```python
from build123d import *

# Parameters (mm, degrees)
F0_R     = 14.2875
F1_DEPTH = 3.175
F2_R     = 8.73125
F3_DEPTH = 1.5875
F5_DEPTH = 1.5875
F6_R     = 7.9375
F6_R_2   = 6.35
F7_DEPTH = 1.5875
F8_COUNT = 6


with BuildPart() as f1:
    # F0 (on Front) → F1 (new body)
    with BuildSketch(Plane.XZ):
        Circle(F0_R)
    extrude(amount=F1_DEPTH)

    # F2 (on face) → F3 (join)
    with BuildSketch(Plane.XZ.offset(3.175)):
        Circle(F2_R)
    extrude(amount=F3_DEPTH)

    # F4 (on face) → F5 (join)
    with BuildSketch(Plane(origin=(0, 0, 0), x_dir=(-1, 0, 0), z_dir=(0, 1, 0))):
        Polygon((11.4293787458, -1.8054905687), (12.8345400717, -0.6283202405), (12.5176613259, 1.1771703282), (10.7956212542, 1.8054905687), (9.3904599283, 0.6283202405), (9.7073386741, -1.1771703282), align=None)
    extrude(amount=F5_DEPTH)

    # F6 (on face) → F7 (join)
    with BuildSketch(Plane(origin=(0, 0, 0), x_dir=(-1, 0, 0), z_dir=(0, 1, 0))):
        Circle(F6_R)
        Circle(F6_R_2, mode=Mode.SUBTRACT)
    extrude(amount=F7_DEPTH)

    # F8: F1 ×6 about axis
    f8_axis = Axis((0, 1.5875, 0), (0, 1, 0))


with BuildPart() as f1_1:
    add(f1.part)
    for i in range(1, F8_COUNT):
        add(f1.part.rotate(f8_axis, i * 360 / F8_COUNT))


solid = f1_1.part
```
Could you check a few things on this model? Use its own coordinates, in mm. A direction names the side the tool comes from. Round coordinates to 2 decimals unless told otherwise and drop trailing zeros. Loops run counter-clockwise (first coordinate to the right, second up) from the corner with the lowest first, then second, coordinate; pieces in that order, holes last. Notation, with made-up numbers: M -25.75,-20.75 L 20.25,-20.75 A21 ccw 20.25,-9.75 Z; hole C 83.5,-35 d7. An arc over 180 degrees is marked long. Put each result on its own line as item: value.
Q1. I need wall thicknesses on probe 1 along Z at (x, y) = (0, 0.85); probe 2 along X at (y, z) = (0.8, 0); probe 3 along Y at (x, z) = (-11.75, 0.75) (1 decimal). Which ranges of each line are inside material? Lowest first, please.
Check result:
probe 1: -7.94 to -6.35, 6.35 to 7.94
probe 2: -12.72 to -9.5, -7.94 to -6.35, 6.35 to 7.94, 9.5 to 12.72
probe 3: -3.2 to 1.6
Q2. Imagine slicing it at C-C (z = 5.5). Write out the boundary of the cut face in (x, y) (1 decimal), then the cut area to 3 significant figures.
Check result:
outline: M -13.2,-3.2 L -6.8,-3.2 L -6.8,-4.8 L 6.8,-4.8 L 6.8,-3.2 L 13.2,-3.2 L 13.2,0 L 5.7,0 L 5.7,1.6 L 3.2,1.6 L 3.2,0 L -3.2,0 L -3.2,1.6 L -5.7,1.6 L -5.7,0 L -13.2,0 Z
area: 113 mm2
Q3. On a 3-axis mill with a long thin cutter (end or side, diameter ignored), from which of +Z, -Z, +X, -X, +Y, -Y can I reach the whole of each face in a straight line? I mean faces 1 (the face through (5, 0.783, -8.137)), 2 (the face through (-7, -3.175, -6)), 3 (the face through (3.99, 0.78, 9.89)), 4 (the face through (10.103, 0.783, -1.225)), 5 (the face through (6.112, 0.783, 8.137)). Say none if no direction works.
Check result:
face 1: +Y
face 2: -Y
face 3: +Z, +Y
face 4: -Z, +Y
face 5: +X, +Y
Q4. For pin 1 (1.5 mm diameter, centred on y = -1, z = -11, fed in from -X); pin 2 (4 mm diameter, centred on x = -0.5, z = 2.5, fed in from +Y), each with a flat end and sliding along its axis, tell me the tip position at first contact or that it passes through.
Check result:
pin 1: x = -9.95
pin 2: y = 0
Q5. Thinking about a two-plate mould opening in X: for faces 6 (the face through (5, 0.78, 11.11)), 7 (the face through (0, -4.762, 0)), 8 (the face through (7.12, 0.78, 9.36)), 9 (the face through (10.56, 0.78, 1.49)), which applies, released by +X, released by -X, zero draft, split by the parting line, or undercut?
Check result:
face 6: undercut
face 7: zero draft
face 8: released by +X
face 9: undercut
Q6. Imagine slicing it at B-B (y = 0.75). State how many separate pieces and enclosed holes the cut face has, then the cut area to 3 significant figures.
Check result:
separate pieces: 7
enclosed holes: 1
area: 124 mm2
